Autodesk Inventor part; units mm, degrees
ref_plane "Work Plane2" through (188.5496, -39.6458, 10.2341) normal (1, 0, 0) x (0, 1, 0)
ref_plane "YZ Plane" through (0, 0, 0) normal (1, 0, 0) x (0, 1, 0)
ref_plane "XZ Plane" through (0, 0, 0) normal (0, 1, 0) x (-1, 0, 0)
ref_plane "Work Plane1" through (89.5496, -22.0458, 63.3377) normal (-1, 0, 0) x (0, -1, 0)
sketch "Sketch1" plane through (89.5496, -22.0458, 63.3377) normal (-1, 0, 0) x (0, -1, 0)
  line L0 (17.6, -19.3036) -> (17.6, 37.9036)
  line L1 (17.6, 37.9036) -> (-22.6, -2.2964)
  line L2 (-22.6, -2.2964) -> (-22.6, -53.1036)
  line L3 (-22.6, -53.1036) -> (-14.1, -53.1036)
  line L4 (-14.1, -53.1036) -> (-14.1, -37.9036)
  arc A0 (4.5, -19.3036) -> (-14.1, -37.9036) centre (4.5, -37.9036) ccw
  line L5 (4.5, -19.3036) -> (17.6, -19.3036)
  line L6 (20.6, 45.1462) -> (20.6, 40.9036)
  line L7 (5.7508, 30.297) -> (20.6, 45.1462)
  line L8 (7.8721, 28.1756) -> (5.7508, 30.297)
  line L9 (20.6, 40.9036) -> (7.8721, 28.1756)
  line L10 (7.8721, 28.1756) -> (6.4579, 29.5899)
  line L11 (6.4579, 29.5899) -> (-23.1664, -0.0344)
  line L12 (-22.6, -2.2964) -> (-23.795, -3.4915)
  line L13 (-23.795, -3.4915) -> (-26.5199, -0.7666)
  line L14 (-23.1664, -0.0344) -> (-26.5411, -3.4091)
  point P0 (-22.0458, -63.3377)
  point P1 (-25.2092, -2.0772)
  dimension "d0" = 2
ref_plane "Work Plane2" through (188.5496, -39.6458, 10.2341) normal (1, 0, 0) x (0, 1, 0)
extrude "Extrusion1" add sketch "Sketch1" against normal up to surface (99 mm away) contours L1 L12 L13 L14 L11 L8
sketch "Sketch2" plane through (89.5496, 3.1634, 61.2604) normal (0, 0.7071, 0.7071) x (1, 0, 0)
  line L0 (99, -44.784) -> (99, 0)
  line L1 (0, 0) -> (99, 0)
  line L2 (0, -44.784) -> (0, 0)
  line L3 (0, -44.784) -> (99, -44.784)
  point P0 (-89.5496, 41.0808)
extrude "Extrusion2" add sketch "Sketch2" along normal blind 1
properties part number "plugg"
Can you work these out from the model? Positions are in its coordinate system, mm. Coordinates: 2 decimals unless noted, no trailing zeros. Loops run counter-clockwise (first coordinate to the right, second up) from the corner with the lowest first, then second, coordinate; pieces in that order, holes last. Notation, with made-up numbers: (-5.75, 78) -> (16.25, 78) arc R13 cw to (16.25, 101) -> close; hole circle Ø9 at (31.5, 3.25). An arc over 180 degrees is marked (long way). Put each result on its own line as item: value. Start each with the question number.
Q1. I'm going to push flat-ended pins straight in: P1, Ø3, axis at x = 141.5, y = -26, coming from the -Z side; P2, Ø5, axis at x = 107.5, y = -6, coming from the +Z side; P3, Ø6, axis at x = 147.5, z = 73.5, coming from the -Y side; P4, Ø3, axis at y = -14.5, z = 84.5, coming from the -X side. Where does each tip first touch, or does it pass through?
Q2. I want a section at B-B (z = 90.5). Write out the boundary of the cut face in (x, y).
Q3. If I drill on line 1 (Z direction, x = 111, y = -21.5); line 2 (Z direction, x = 121, y = -4.5); line 3 (Y direction, x = 167, z = 81), over which ranges is the centre line in solid material (lowest first)? Write a range as [from, to].
Q4. I want a section at C-C (y = -24.5). Write out the boundary of the cut face in (x, z), plus the area to 3 significant figures.
Taken from the geometry:
1. P1: stops at z = 86.1
1. P2: stops at z = 74.34
1. P3: stops at y = -14.9
1. P4: passes through
2. outline: (89.55, -28.9) -> (188.55, -28.9) -> (188.55, -24.66) -> (89.55, -24.66) -> close
3. line 1: z = [83.1, 87.34]
3. line 2: z = [66.1, 70.34]
3. line 3: y = [-19.4, -15.16]
4. outline: (89.55, 86.1) -> (188.55, 86.1) -> (188.55, 90.34) -> (89.55, 90.34) -> close
4. area: 420 mm2
